Autodesk Inventor part; units mm, degrees
ref_plane "YZ Plane" through (0, 0, 0) normal (1, 0, 0) x (0, 1, 0)
ref_plane "XZ Plane" through (0, 0, 0) normal (0, 1, 0) x (-1, 0, 0)
ref_plane "XY Plane" through (0, 0, 0) normal (0, 0, 1) x (1, 0, 0)
sketch "Sketch1" plane through (0, 0, 0) normal (0, 1, 0) x (-1, 0, 0)
  line L0 (0, 279.3478) -> (-39.1304, 279.3478)
  line L1 (-39.1304, 279.3478) -> (-39.1304, -195.6522)
  line L2 (-39.1304, -195.6522) -> (0, -195.6522)
  line L3 (0, -195.6522) -> (0, 279.3478)
  line L4 (-39.1304, 279.3478) -> (-29.1304, 279.3478)
  line L5 (-29.1304, 254.3478) -> (-39.1304, 254.3478)
  line L6 (-39.1304, 254.3478) -> (-39.1304, 279.3478)
  line L7 (-39.1304, -195.6522) -> (-29.1304, -195.6522)
  line L8 (-29.1304, -170.6522) -> (-39.1304, -170.6522)
  line L9 (-39.1304, -170.6522) -> (-39.1304, -195.6522)
  point P0 (0, 0)
  point P1 (-39.1304, 254.3478)
  dimension "d0" = 475
  dimension "d4" = 25
  dimension "d5" = 25
extrude "Extrusion1" add sketch "Sketch1" along normal blind 160
sketch "Sketch2" plane through (0, 0, 279.3478) normal (0, 0, 1) x (1, 0, 0)
  line L0 (0, 160) -> (39.1304, 160)
  line L1 (0, 160) -> (39.1304, 160)
  line L2 (39.1304, 160) -> (39.1304, 0)
  line L3 (39.1304, 0) -> (0, 0)
  line L4 (0, 0) -> (0, 160)
  line L5 (39.1304, 160) -> (29.1304, 160)
  line L6 (29.1304, 160) -> (29.1304, 115)
  line L7 (29.1304, 115) -> (39.1304, 115)
  line L8 (39.1304, 115) -> (39.1304, 160)
  line L9 (39.1304, 0) -> (29.1304, 0)
  line L10 (29.1304, 0) -> (29.1304, 45)
  line L11 (29.1304, 45) -> (39.1304, 45)
  line L12 (39.1304, 45) -> (39.1304, 0)
  circle A0 centre (39.1304, 80) radius 18
  line L13 (35.1304, 75) -> (39.1304, 75)
  line L14 (39.1304, 75) -> (39.1304, 98)
  line L15 (39.1304, 98) -> (35.1304, 98)
  line L16 (35.1304, 98) -> (35.1304, 75)
  line L17 (35.1304, 75) -> (39.1304, 75)
  line L18 (39.1304, 75) -> (39.1304, 62)
  line L19 (39.1304, 62) -> (35.1304, 62)
  line L20 (35.1304, 62) -> (35.1304, 75)
  line L21 (39.1304, 0) -> (39.1304, 160)
  line L22 (0, 160) -> (19.1304, 160)
  line L23 (19.1304, 160) -> (19.1304, 0)
  line L24 (19.1304, 0) -> (0, 0)
  line L25 (0, 0) -> (0, 160)
  point P0 (0, 0)
  point P1 (34.1304, 115)
  point P2 (34.1304, 160)
  point P3 (39.1304, 45)
  point P4 (39.1304, 115)
  dimension "d6" = 10
  dimension "d7" = 45
  dimension "d8" = 45
  dimension "d9" = 4
  dimension "d10" = 36
  dimension "d11" = 80
  dimension "d12" = 80
  dimension "d15" = 20
extrude "Extrusion2" cut sketch "Sketch2" against normal up to surface (475 mm away) contours L0 L23 L3 L4 | L0 L2 L7 L6 | L10 L11 L2 L3 | L2 L13 L16 A0 | A0 L16 L15 | L2 A0 L20 L13 | L19 L20 A0
sketch "Sketch3" plane through (0, 160, 0) normal (0, 1, 0) x (1, 0, 0)
  line L0 (-18, 249) -> (160, 249)
  line L1 (160, 249) -> (160, 90.6522)
  line L2 (160, 90.6522) -> (-18, 90.6522)
  line L3 (-18, 90.6522) -> (-18, 249)
  line L4 (19.1304, -279.3478) -> (29.1304, -279.3478)
  point P0 (0, 0)
  dimension "d16" = 370
extrude "Extrusion3" cut sketch "Sketch3" against normal blind 200
sketch "Sketch4" plane through (39.1304, 98, 279.3478) normal (1, 0, 0) x (0, 0, -1)
  line L0 (370, 0) -> (370, 17)
  line L1 (370, 17) -> (0, 17)
  line L2 (0, 0) -> (0, 17)
  line L3 (0, 0) -> (370, 0)
  line L4 (370, -53) -> (370, -36)
  line L5 (370, -36) -> (0, -36)
  line L6 (0, -53) -> (0, -36)
  line L7 (0, -53) -> (370, -53)
  point P0 (279.3478, -98)
extrude "Extrusion4" add sketch "Sketch4" along normal blind 30
sketch "Sketch5" plane through (19.1304, 0, 279.3478) normal (-1, 0, 0) x (0, 0, 1)
  line L0 (-370, 160) -> (-370, 0)
  line L1 (0, 0) -> (-370, 0)
  line L2 (0, 160) -> (0, 0)
  line L3 (-370, 160) -> (0, 160)
  point P0 (-279.3478, 0)
extrude "Extrusion5" add sketch "Sketch5" along normal blind 5
sketch "Sketch6" plane through (29.1304, 115, 279.3478) normal (0, 0, 1) x (1, 0, 0)
  line L0 (9, 13) -> (-3, 13)
  line L1 (-3, 13) -> (-3, 45)
  line L2 (-3, 45) -> (9, 45)
  line L3 (9, 45) -> (9, 13)
  line L4 (-15, -115) -> (0, -115)
  line L5 (11, -83) -> (-3, -83)
  line L6 (-3, -83) -> (-3, -115)
  line L7 (-3, -115) -> (11, -115)
  line L8 (11, -115) -> (11, -83)
  line L9 (0, -70) -> (40, -70)
  line L10 (0, 0) -> (40, 0)
  line L11 (0, 0) -> (0, 45)
  point P0 (-29.1304, -115)
  point P1 (0, -115)
  dimension "d23" = 13
  dimension "d24" = 13
  dimension "d25" = 3
extrude "Extrusion6" cut sketch "Sketch6" against normal blind 500
sketch "Sketch7" plane through (35.1304, 62, 279.3478) normal (0, 0, 1) x (1, 0, 0)
  line L0 (55, 54) -> (-8, 54)
  line L1 (-8, 54) -> (-8, -18)
  line L2 (-8, -18) -> (55, -18)
  line L3 (55, -18) -> (55, 54)
  line L4 (-6, 53) -> (34, 53)
  line L5 (-6, -17) -> (34, -17)
  line L6 (-6, -30) -> (-6, -17)
  point P0 (-35.1304, -62)
  dimension "d28" = 1
  dimension "d29" = 1
  dimension "d30" = 2
extrude "Extrusion7" cut sketch "Sketch7" against normal blind 1000
properties part number "MainRails" material "Aluminum 6061"
Geometry check sheet. Reference: the model listing, model coordinates, mm. A direction names the side the tool comes from. Round coordinates to 2 decimals unless told otherwise and drop trailing zeros. Loops run counter-clockwise (first coordinate to the right, second up) from the corner with the lowest first, then second, coordinate; pieces in that order, holes last. Notation, with made-up numbers: M 33.25,52 L 66.25,52 A20 cw 66.25,89 Z; hole C 64.25,22.5 d11. An arc over 180 degrees is marked long. Return JSON: item names as keys, results as strings. Group by question number.
(1) Go/stop test with flat-tipped pins: pin 1 (16 mm diameter, centred on y = 149, z = 75.5, fed in from +X); pin 2 (2 mm diameter, centred on x = 28, z = 3, fed in from -Y); pin 3 (0.6 mm diameter, centred on x = 28, z = 99.5, fed in from +Y). Record where each tip stops, or that it passes through.
(2) Section check A-A, the plane z = 163.5. Enter the section's corners in (x, y), and give its area (3 significant figures).
(3) Set-up check for faces 1 (the face through (26.13, 16, 97)), 2 (the face through (29.13, 122, 97)), 3 (the face through (26.13, 144, 97)): record each of +Z, -Z, +X, -X, +Y, -Y from which the full face is reachable in a straight line by a thin tool's end or side.
(4) Scan lines: line 1 along X through (y, z) = (68, -60); line 2 along X through (y, z) = (22.5, 258); line 3 along Y through (x, z) = (26.5, 79). Record each from-to range of solid material in increasing order. Write a range as [from, to].
(5) Mould release check, pull along Y, two halves, no side actions. Record for faces 4 (the face through (20, 81, -90.652)), 5 (the face through (20, 0, 97)), 6 (the face through (20, 160, 92)), 7 (the face through (27.13, 81, 97)): pulls with the +Y half, pulls with the -Y half, needs draft (parallel to the pull), parting line crosses it, or undercut.
(6) Section check B-B, the plane y = 15. Enter the section's corners in (x, z), and give its area (3 significant figures).
(7) Section check C-C, the plane y = 70. Enter the section's corners in (x, z).
Data:
{
 "1": {"pin 1": "x = 26.13", "pin 2": "y = 32", "pin 3": "y = 128"},
 "2": {"outline": "M 14.13,0 L 26.13,0 L 26.13,32 L 29.13,32 L 29.13,44 L 27.13,44 L 27.13,116 L 29.13,116 L 29.13,128 L 26.13,128 L 26.13,160 L 14.13,160 Z", "area": "2,060 mm²"},
 "3": {"face 1": "+Z, -Z, +X, -Y", "face 2": "+Z, -Z, +X, +Y, -Y", "face 3": "+Z, -Z, +X, +Y"},
 "4": {"line 1": "[14.13, 27.13]", "line 2": "[14.13, 26.13]", "line 3": "[32, 128]"},
 "5": {"face 4": "needs draft", "face 5": "pulls with the -Y half", "face 6": "pulls with the +Y half", "face 7": "undercut"},
 "6": {"outline": "M 14.13,-90.65 L 26.13,-90.65 L 26.13,279.35 L 14.13,279.35 Z", "area": "4,440 mm²"},
 "7": {"outline": "M 14.13,-90.65 L 27.13,-90.65 L 27.13,279.35 L 14.13,279.35 Z"}
}
